from build123d import *

# Parameters (mm, degrees)
BOSS_EXTRUDE1_DEPTH      = 5
BOSS_EXTRUDE1_DEPTH_BACK = 563.8
CUT_EXTRUDE1_DEPTH       = 7.42512
BOSS_EXTRUDE2_DEPTH      = 91.3
SKETCH4_R                = 0.69
SKETCH4_R_2              = 0.51
CUT_EXTRUDE2_DEPTH       = 2
SKETCH5_R                = 1
CUT_EXTRUDE3_DEPTH       = 7.42512


with BuildPart() as part:
    # Sketch1 → Boss-Extrude1 (new body, two sides)
    with BuildSketch(Plane(origin=(0, 0, 0), x_dir=(0, 0, -1), z_dir=(1, 0, 0))) as boss_extrude1_sk:
        with BuildLine():
            Line((0, 0), (-61, 0))
            ThreePointArc((-61, 0), (-64.21256, -3.21256), (-61, -6.42512))
            Line((-61, -6.42512), (0, -6.42512))
            Line((0, -6.42512), (5, -6.42512))
            Line((5, -6.42512), (5, -6.26256))
            Line((5, -6.26256), (-61, -6.26256))
            ThreePointArc((-61, -6.26256), (-64.05, -3.21256), (-61, -0.16256))
            Line((-61, -0.16256), (5, -0.16256))
            Line((5, -0.16256), (5, 0))
            Line((5, 0), (0, 0))
        make_face()
    extrude(amount=BOSS_EXTRUDE1_DEPTH)
    extrude(boss_extrude1_sk.sketch, amount=-BOSS_EXTRUDE1_DEPTH_BACK)

    # Sketch2 → Cut-Extrude1 (cut, through all)
    with BuildSketch(Plane(origin=(0, 0, 0), x_dir=(1, 0, 0), z_dir=(0, 1, 0))):
        with BuildLine():
            Line((5, 0), (1, 0))
            ThreePointArc((1, 0), (0.292893219, 0.292893219), (0, 1))
            Line((0, 1), (0, 5))
            Line((0, 5), (-5, 5))
            Line((-5, 5), (-5, 1))
            ThreePointArc((-5, 1), (-5.292893219, 0.292893219), (-6, 0))
            Line((-6, 0), (-457.8, 0))
            ThreePointArc((-457.8, 0), (-458.507106781, 0.292893219), (-458.8, 1))
            Line((-458.8, 1), (-458.8, 5))
            Line((-458.8, 5), (-463.8, 5))
            Line((-463.8, 5), (-463.8, 1))
            ThreePointArc((-463.8, 1), (-464.092893219, 0.292893219), (-464.8, 0))
            Line((-464.8, 0), (-563.8, 0))
            Line((-563.8, 0), (-563.8, 10))
            Line((-563.8, 10), (5, 10))
            Line((5, 10), (5, 0))
        make_face()
    extrude(amount=-CUT_EXTRUDE1_DEPTH, mode=Mode.SUBTRACT)

    # Sketch3 → Boss-Extrude2 (add)
    with BuildSketch(Plane.ZY.offset(563.8)):
        with BuildLine():
            Line((61, -0.23114), (0, -0.23114))
            Line((0, -0.23114), (0, 0))
            Line((0, 0), (61, 0))
            ThreePointArc((61, 0), (64.21256, -3.21256), (61, -6.42512))
            Line((61, -6.42512), (0, -6.42512))
            Line((0, -6.42512), (0, -6.19398))
            Line((0, -6.19398), (61, -6.19398))
            ThreePointArc((61, -6.19398), (63.98142, -3.21256), (61, -0.23114))
        make_face()
    extrude(amount=-BOSS_EXTRUDE2_DEPTH)

    # Sketch4 → Cut-Extrude2 (cut)
    with BuildSketch(Plane(origin=(0, 0, 0), x_dir=(1, 0, 0), z_dir=(0, 1, 0))):
        with Locations(Location((-560.001, -43.918, 0), (0, 0, 270))):  # turned: the seam where the file's is
            Circle(SKETCH4_R)
        with Locations(Location((-534.001, -43.918, 0), (0, 0, 270))):  # turned: the seam where the file's is
            Circle(SKETCH4_R_2)
        with Locations(Location((-531.001, -50.418, 0), (0, 0, 270))):  # turned: the seam where the file's is
            Circle(SKETCH4_R)
        with Locations(Location((-505.001, -50.418, 0), (0, 0, 270))):  # turned: the seam where the file's is
            Circle(SKETCH4_R_2)
        with Locations(Location((-502.001, -56.918, 0), (0, 0, 270))):  # turned: the seam where the file's is
            Circle(SKETCH4_R)
        with Locations(Location((-476.001, -56.918, 0), (0, 0, 270))):  # turned: the seam where the file's is
            Circle(SKETCH4_R_2)
    extrude(amount=-CUT_EXTRUDE2_DEPTH, mode=Mode.SUBTRACT)

    # Sketch5 → Cut-Extrude3 (cut, through all)
    with BuildSketch(Plane(origin=(0, 0, 0), x_dir=(1, 0, 0), z_dir=(0, 1, 0))):
        with Locations(Location((-460.8, 2.99, 0), (0, 0, 270))):  # turned: the seam where the file's is
            Circle(SKETCH5_R)
        with Locations(Location((-2, 2.99, 0), (0, 0, 270))):  # turned: the seam where the file's is
            Circle(SKETCH5_R)
    extrude(amount=-CUT_EXTRUDE3_DEPTH, mode=Mode.SUBTRACT)


solid = part.part
Read the model definition and answer for the solid it produces. Units are mm, in the model's axes. Give positions to 0.01 mm unless a question says otherwise; leave off trailing zeros. Loops run counter-clockwise (first coordinate to the right, second up) from the corner with the lowest first, then second, coordinate; pieces in that order, holes last. Notation, with made-up numbers: (29.5, 25.25) - (72.5, 25.25) arc R29 ccw to (72.5, 59.25) - close; hole circle Ø7 at (77, 69). An arc over 180 degrees is marked (long way). Answer as CSV lines item,"result". Start each with the question number.
1) Each of these flat-tipped pins is pushed along its axis until it touches: pin 1 Ø0.9 at (x, z) = (-505.001, 50.418) entering from +Y; pin 2 Ø1.8 at (x, z) = (-460.8, -2.99) entering from +Y; pin 3 Ø1 at (x, y) = (-353.5, -4) entering from -Z. Where does it stop, or does it pass through?
2) Determine the mould class of faces 1 (the face through (-230, -0.163, 36)), 2 (the face through (-275, -6.425, 36)), 3 (the face through (-275, 0, 35)) for opening direction Y: released by +Y, released by -Y, zero draft, split by the parting line, or undercut.
3) Find section A-A (z = 32). Write down the section's boundary in (x, y).
4) Find section B-B (x = -172.5). Write down the section's boundary in (y, z).
5) Straight lines are drawn through the part: L1, parallel to X at y = -6.3, z = -2.99; L2, parallel to Y at x = -457.5, z = 24.5; L3, parallel to Y at x = -522.5, z = 17. For each, find the intervals that lie inside material, in ascending order. Write a range as from..to.
6) Find section C-C (y = -3). Write down the section's boundary in (x, z), then the cut area to 3 significant figures.
Findings below:
1,pin 1,"y = -6.19"
1,pin 2,"through"
1,pin 3,"z = 63.76"
2,face 1,"undercut"
2,face 2,"released by -Y"
2,face 3,"released by +Y"
3,outline,"(-563.8, -6.43) - (5, -6.43) - (5, -6.26) - (-472.5, -6.26) - (-472.5, -6.19) - (-563.8, -6.19) - close; (-563.8, -0.23) - (-472.5, -0.23) - (-472.5, -0.16) - (5, -0.16) - (5, 0) - (-563.8, 0) - close"
4,outline,"(-6.43, 0) - (-6.26, 0) - (-6.26, 61) arc R3.05 cw to (-0.16, 61) - (-0.16, 0) - (0, 0) - (0, 61) arc R3.21 ccw to (-6.43, 61) - close"
5,L1,"-463.8..-461.8, -459.8..-458.8, -5..-3, -1..0"
5,L2,"-6.43..-6.26, -0.16..0"
5,L3,"-6.43..-6.19, -0.23..0"
6,outline,"(-563.8, 63.97) - (-472.5, 63.97) - (-472.5, 64.04) - (5, 64.04) - (5, 64.21) - (-563.8, 64.21) - close"
6,area,"99.0 mm^2"
